For this review, take the finished solid that the model builds, in its own axes (mm). Face numbers are marked on the shaded views. A direction names the side the tool comes from. Round coordinates to 2 decimals unless told otherwise and drop trailing zeros. Write each loop counter-clockwise with the first axis right and the second up, starting at its lowest first coordinate (ties: lowest second). Pieces come first, ordered by that corner, then holes. Notation, with made-up numbers: (61.5, 78) -> (98.5, 78) arc R23 cw to (98.5, 92) -> close; hole circle Ø4 at (-17, 71.5). An arc over 180 degrees is marked (long way). Write item = value, one per line. Start each with the question number.
```python
from build123d import *

# Parameters (mm, degrees)
SKETCH1_R           = 12.15
BOSS_EXTRUDE1_DEPTH = 50
SKETCH2_R           = 3.5
BOSS_EXTRUDE2_DEPTH = 2.5
BOSS_EXTRUDE3_DEPTH = 9.5
SKETCH4_R           = 1.901379474
BOSS_EXTRUDE4_DEPTH = 1.5


with BuildPart() as part:
    # Sketch1 → Boss-Extrude1 (new body)
    with BuildSketch(Plane(origin=(0, 0, 0), x_dir=(1, 0, 0), z_dir=(0, 1, 0))):
        Circle(SKETCH1_R)
    extrude(amount=BOSS_EXTRUDE1_DEPTH)

    # Sketch2 → Boss-Extrude2 (add)
    with BuildSketch(Plane(origin=(0, 50, 0), x_dir=(1, 0, 0), z_dir=(0, 1, 0))):
        Circle(SKETCH2_R)
    extrude(amount=BOSS_EXTRUDE2_DEPTH)

    # Sketch3 → Boss-Extrude3 (add)
    with BuildSketch(Plane(origin=(0, 52.5, 0), x_dir=(1, 0, 0), z_dir=(0, 1, 0))):
        with BuildLine():
            Line((-1.598620526, 1.029396092), (-1.598620526, -1.029396092))
            ThreePointArc((-1.598620526, -1.029396092), (1.901379474, 0), (-1.598620526, 1.029396092))
        make_face()
    extrude(amount=BOSS_EXTRUDE3_DEPTH)

    # Sketch4 → Boss-Extrude4 (add)
    with BuildSketch(Plane(origin=(0, 52.5, 0), x_dir=(1, 0, 0), z_dir=(0, 1, 0))):
        Circle(SKETCH4_R)
    extrude(amount=BOSS_EXTRUDE4_DEPTH)


solid = part.part
```
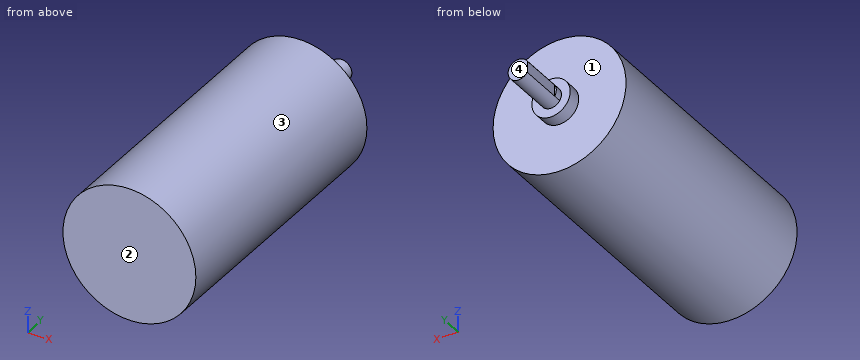
1. Wall thickness on L1, parallel to Y at x = 1, z = 9; L2, parallel to X at y = 37.5, z = 0.5; L3, parallel to X at y = 25, z = 10: over which ranges is each line inside the solid? List them lowest first. Write a range as from..to.
2. Consider section D-D, the plane y = 16. Give the boundary of the cut face in (x, z).
3. Machinability: for the marked faces 1 and 2, which of the approach directions +Z, -Z, +X, -X, +Y, -Y give a long, thin tool a straight path to every point of the face, cutting with its end or side? Answer none if there is none.
4. Consider section B-B, the plane z = 0. Give the boundary of the cut face in (x, y), then the cut area to 3 significant figures.
5. Consider section C-C, the plane y = 51. Give the boundary of the cut face in (x, z), then the cut area to 3 significant figures.
6. Clearance check with flat-ended pins moving along their axes: pin 1 Ø6 at (y, z) = (49, 4) entering from +X; pin 2 Ø10 at (x, y) = (-5.5, 49.5) entering from +Z; pin 3 Ø1.6 at (y, z) = (56.5, 0) entering from -X. State where each tip first meets the part, or that it passes through.
7. Draft analysis for pull direction X (two halves, no side actions). For the marked faces 3 and 4, state which applies: +X half, -X half, draft (parallel to the pull), parting line (faces both ways), or undercut.
8. Consider section A-A, the plane x = 0. Give the boundary of the cut face in (y, z).
Outcome:
q1.L1 = 0..50
q1.L2 = -12.14..12.14
q1.L3 = -6.9..6.9
q2.outline = circle Ø24.3 at (0, 0)
q3.face_1 = +Y
q3.face_2 = +Z, -Z, +X, -X, -Y
q4.outline = (-12.15, 0) -> (12.15, 0) -> (12.15, 50) -> (3.5, 50) -> (3.5, 52.5) -> (1.9, 52.5) -> (1.9, 62) -> (-1.6, 62) -> (-1.6, 54) -> (-1.9, 54) -> (-1.9, 52.5) -> (-3.5, 52.5) -> (-3.5, 50) -> (-12.15, 50) -> close
q4.area = 1,270 mm2
q5.outline = circle Ø7 at (0, 0)
q5.area = 38.5 mm2
q6.pin_1 = 12.11
q6.pin_2 = 12.14
q6.pin_3 = -1.6
q7.face_3 = parting line
q7.face_4 = draft
q8.outline = (0, -12.15) -> (50, -12.15) -> (50, -3.5) -> (52.5, -3.5) -> (52.5, -1.9) -> (62, -1.9) -> (62, 1.9) -> (52.5, 1.9) -> (52.5, 3.5) -> (50, 3.5) -> (50, 12.15) -> (0, 12.15) -> close
